The listing builds one solid part. Answer for the finished solid, in the listing's coordinates (mm). Face numbers are marked on the shaded views. Round coordinates to 2 decimals unless told otherwise and drop trailing zeros. Order: outer loops, then holes, each group sorted by start corner. A loop starts at its lowest first (then second) coordinate and runs counter-clockwise, first axis right, second up. Notation, with made-up numbers: M -39.75,65 L -27.75,65 A26 cw -27.75,90 Z; hole C 68.25,-12.75 d1. An arc over 180 degrees is marked long. Write item = value, one per line. Start each with the question number.
(1) Straight lines are drawn through the part: probe 1 along Z at (x, y) = (0.5, 0) (3 decimals); probe 2 along Z at (x, y) = (-10.75, 2.5); probe 3 along Z at (x, y) = (-2.5, -2.5). For each, find the intervals that lie inside material, in ascending order. Write a range as from..to.
(2) Each of these flat-tipped pins is pushed along its axis until it touches: pin 1 (4 mm diameter, centred on x = 9.5, z = 7, fed in from +Y); pin 2 (4 mm diameter, centred on y = -4, z = 14, fed in from +X) (3 decimals); pin 3 (1.2 mm diameter, centred on x = -1.5, z = 1.5, fed in from +Y); pin 4 (5 mm diameter, centred on y = -2.5, z = 10.5, fed in from +X). Where does it stop, or does it pass through?
(3) A cutting plane is placed at B-B, the plane y = 0. Determine the outline of the cut face in (x, z) (3 decimals), and give its area (3 significant figures).
(4) For a pull along Y with two mould halves and no side action, classify the marked faces 1, 2, 3 and 4 as released by +Y, released by -Y, zero draft, split by the parting line, or undercut.
from build123d import *

# Parameters (mm, degrees)
F0_W     = 26.9875
F0_H     = 15.875
F1_DEPTH = 2.38125
F2_R     = 6.35
F3_DEPTH = 9.525


# Not quite as in the source:
# - a fillet or chamfer that OpenCascade refuses, or shapes differently, is made with other operations: its cross-section is extruded or revolved along the edge and cut away or added


with BuildPart() as f1:
    # F0 (on Top) → F1 (new body)
    with BuildSketch(Plane.XY):
        Rectangle(F0_W, F0_H)
    extrude(amount=F1_DEPTH)

    # F2 (on Right) → F3 (join, symmetric)
    with BuildSketch(Plane.YZ):
        with BuildLine():
            ThreePointArc((5.0201157855, 2.38125), (7.7481163038, 5.4999012055), (8.73125, 9.525))
            ThreePointArc((8.73125, 9.525), (-4.0250987945, 17.2731163038), (-5.0201157855, 2.38125))
            Line((-5.0201157855, 2.38125), (5.0201157855, 2.38125))
        make_face()
        with Locations((0, 9.525)):
            Circle(F2_R, mode=Mode.SUBTRACT)
    extrude(amount=F3_DEPTH, both=True)

    # F4: chamfer of 1.27 on 2 edges, made by hand


with BuildPart() as f4_tool2:
    # F4_s3 → F4_t4 (revolve)
    with BuildSketch(Plane.XY.offset(9.525)):
        Polygon((9.525, 7.62), (8.255, 6.35), (9.525, 6.35), align=None)
    revolve(axis=Axis((9.525, 0, 9.525), (1, 0, 0)))

    split(bisect_by=Plane.XY.offset(2.38125), keep=Keep.TOP)


with BuildPart() as f1_1:
    add(f1.part)

    # F4_t1: cut F4_tool2
    add(f4_tool2.part, mode=Mode.SUBTRACT)


with BuildPart() as f4_tool7:
    # F4_s8 → F4_t9 (revolve)
    with BuildSketch(Plane.XY.offset(9.525)):
        Polygon((-9.525, 7.62), (-8.255, 6.35), (-9.525, 6.35), align=None)
    revolve(axis=Axis((-9.525, 0, 9.525), (1, 0, 0)))

    split(bisect_by=Plane.XY.offset(2.38125), keep=Keep.TOP)


with BuildPart() as f1_2:
    add(f1_1.part)

    # F4_t6: cut F4_tool7
    add(f4_tool7.part, mode=Mode.SUBTRACT)


solid = f1_2.part
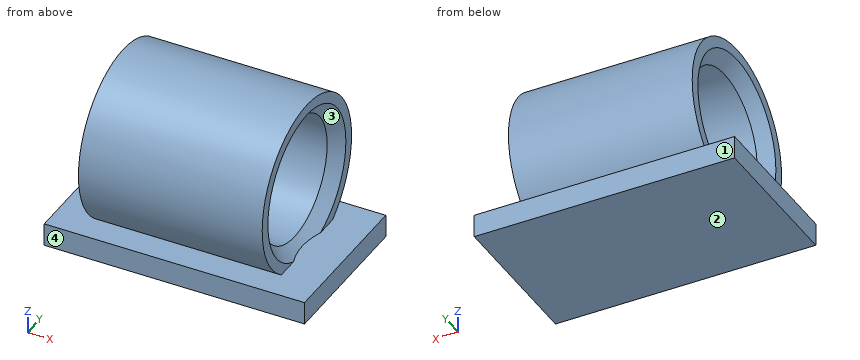
Reported:
q1.probe_1 = 0..3.175, 15.875..18.256
q1.probe_2 = 0..2.38
q1.probe_3 = 0..3.69, 15.36..17.89
q2.pin_1 = 8.72
q2.pin_2 = 9.525
q2.pin_3 = 7.94
q2.pin_4 = through
q3.outline = M -13.494,0 L 13.494,0 L 13.494,2.381 L 9.049,2.381 L 8.255,3.175 L -8.255,3.175 L -9.049,2.381 L -13.494,2.381 Z; M -9.525,17.145 L -8.255,15.875 L 8.255,15.875 L 9.525,17.145 L 9.525,18.256 L -9.525,18.256 Z
q3.area = 122 mm²
q4.face_1 = released by +Y
q4.face_2 = zero draft
q4.face_3 = undercut
q4.face_4 = released by -Y
